from build123d import *

# Parameters (mm, degrees)
SKETCH1_R           = 11.1379
BOSS_EXTRUDE1_DEPTH = 3.7465
SKETCH2_R           = 5.1181
BOSS_EXTRUDE2_DEPTH = 8.9281
SKETCH3_R           = 5.1181
BOSS_EXTRUDE3_DEPTH = 2.54
SKETCH4_R           = 3.9751
CUT_EXTRUDE1_DEPTH  = 16.2146
SKETCH5_R           = 1.7526
CUT_EXTRUDE2_DEPTH  = 13.6746


with BuildPart() as part:
    # Sketch1 → Boss-Extrude1 (new body)
    with BuildSketch(Plane.XY):
        Circle(SKETCH1_R)
    extrude(amount=BOSS_EXTRUDE1_DEPTH)

    # Sketch2 → Boss-Extrude2 (add)
    with BuildSketch(Plane(origin=(0, 0, 0), x_dir=(-1, 0, 0), z_dir=(0, 0, -1))):
        Circle(SKETCH2_R)
    extrude(amount=BOSS_EXTRUDE2_DEPTH)

    # Sketch3 → Boss-Extrude3 (add)
    with BuildSketch(Plane.XY.offset(3.7465)):
        Circle(SKETCH3_R)
    extrude(amount=BOSS_EXTRUDE3_DEPTH)

    # Sketch4 → Cut-Extrude1 (cut, through all)
    with BuildSketch(Plane(origin=(0, 0, -8.9281), x_dir=(-1, 0, 0), z_dir=(0, 0, -1))):
        Circle(SKETCH4_R)
    extrude(amount=-CUT_EXTRUDE1_DEPTH, mode=Mode.SUBTRACT)

    # Sketch5 → Cut-Extrude2 (cut, through all)
    with BuildSketch(Plane.XY.offset(3.7465)):
        with Locations((0, 8.5979)):
            Circle(SKETCH5_R)
        with Locations((8.5979, 0)):
            Circle(SKETCH5_R)
        with Locations((0, -8.5979)):
            Circle(SKETCH5_R)
        with Locations((-8.5979, 0)):
            Circle(SKETCH5_R)
    extrude(amount=-CUT_EXTRUDE2_DEPTH, mode=Mode.SUBTRACT)


solid = part.part
Design review of the part built by this model. Coordinates are the model's own, in mm. A direction names the side the tool comes from. Coordinates: 2 decimals unless noted, no trailing zeros. Loops run counter-clockwise (first coordinate to the right, second up) from the corner with the lowest first, then second, coordinate; pieces in that order, holes last.
Item 1: Add section C-C (y = 9). Write out the cut boundary in (x, z).
Completed:
outline: (-6.56, 0) - (-1.71, 0) - (-1.71, 3.75) - (-6.56, 3.75) - close; (1.71, 0) - (6.56, 0) - (6.56, 3.75) - (1.71, 3.75) - close
Item 2: Add section A-A (x = 0). Write out the cut boundary in (y, z).
Completed:
outline: (-11.14, 0) - (-10.35, 0) - (-10.35, 3.75) - (-11.14, 3.75) - close; (-6.85, 0) - (-5.12, 0) - (-5.12, -8.93) - (-3.98, -8.93) - (-3.98, 6.29) - (-5.12, 6.29) - (-5.12, 3.75) - (-6.85, 3.75) - close; (3.98, -8.93) - (5.12, -8.93) - (5.12, 0) - (6.85, 0) - (6.85, 3.75) - (5.12, 3.75) - (5.12, 6.29) - (3.98, 6.29) - close; (10.35, 0) - (11.14, 0) - (11.14, 3.75) - (10.35, 3.75) - close
Item 3: Add section D-D (z = -5.75). Write out the cut boundary in (x, y).
Completed:
outline: circle Ø10.24 at (0, 0); hole circle Ø7.95 at (0, 0)
Item 4: Clearance check with flat-ended pins moving along their axes: pin 1 (4 mm diameter, centred on x = 5.5, z = 0, fed in from +Y); pin 2 (1 mm diameter, centred on y = 7, z = 0.5, fed in from +X); pin 3 (3 mm diameter, centred on x = 9, y = -1.5, fed in from +Z); pin 4 (1.5 mm diameter, centred on x = 8, z = -1, fed in from +Y). State where each tip first meets the part, or that it passes through.
Completed:
pin 1: stops at y = 10.57
pin 2: stops at x = 9.04
pin 3: stops at z = 3.75
pin 4: passes through
Item 5: Draft analysis for pull direction X (two halves, no side actions). For faces 1 (the cylindrical face through (-1.45, 11.043, 1.847)), 2 (the cylindrical face through (-0.23, -6.86, 1.9)), 3 (the flat face through (3, -3, 6.286)), state which applies: pulls with the +X half, pulls with the -X half, needs draft (parallel to the pull), parting line crosses it, or undercut.
Completed:
face 1: parting line crosses it
face 2: undercut
face 3: needs draft
Item 6: For faces 4 (the flat face through (5, -2, 3.746)), 5 (the cylindrical face through (5.113, 0.225, -4.402)), 6 (the cylindrical face through (10.27, 0.53, 1.9)), list the 3-axis set-ups (+Z, -Z, +X, -X, +Y, -Y) from which the entire face can be reached by the end or side of a thin tool; tool diameter is ignored.
Completed:
face 4: +Z
face 5: -Z
face 6: +Z, -Z
Item 7: Wall thickness on L1, parallel to Y at x = 0, z = 2.5; L2, parallel to Y at x = 2.75, z = -7.75; L3, parallel to X at y = 1.25, z = 0.75: over which ranges is each line inside the solid? List them lowest first.
Completed:
L1: y = -11.14 to -10.35, -6.85 to -3.98, 3.98 to 6.85, 10.35 to 11.14
L2: y = -4.32 to -2.87, 2.87 to 4.32
L3: x = -11.07 to -9.83, -7.37 to -3.77, 3.77 to 7.37, 9.83 to 11.07
